```python
from build123d import *

# Parameters (mm, degrees)
SKETCH1_W          = 80
SKETCH1_H          = 15
SHELL2_T           = 1
SKETCH2_R          = 1
CUT_EXTRUDE1_DEPTH = 10
FILLET1_R          = 2


with BuildPart() as part:
    # Sketch1 → Revolve1 (revolve)
    with BuildSketch(Plane.XY, mode=Mode.PRIVATE) as revolve1_sk:
        with Locations((40, 7.5)):
            Rectangle(SKETCH1_W, SKETCH1_H)
    revolve(revolve1_sk.sketch.rotate(Axis((0, 0, 0), (1, 0, 0)), 90), axis=Axis((0, 0, 0), (1, 0, 0)))

    # Shell2 (no face opened: a closed hollow body)
    add(offset(amount=-SHELL2_T, mode=Mode.PRIVATE), mode=Mode.SUBTRACT)

    # Sketch2 → Cut-Extrude1 (cut)
    with BuildSketch(Plane(origin=(80, 0, 0), x_dir=(0, 0, -1), z_dir=(1, 0, 0))):
        Circle(SKETCH2_R)
    extrude(amount=-CUT_EXTRUDE1_DEPTH, mode=Mode.SUBTRACT)

    # Fillet1
    fillet1_edges = [part.edges().sort_by_distance(p)[0] for p in [
        (0, 0, -15),
        (80, 0, -15),
    ]]
    fillet(fillet1_edges, radius=FILLET1_R)


solid = part.part
```
CAD build for the part. Positions are in the model's coordinates, mm. A direction names the side the tool comes from. Coordinates: 2 decimals unless noted, no trailing zeros. Order: outer loops, then holes, each group sorted by start corner. A loop starts at its lowest first (then second) coordinate and runs counter-clockwise, first axis right, second up. Notation, with made-up numbers: (83.25, -39) - (139.25, -39) arc R24 ccw to (139.25, -22) - close; hole circle Ø8 at (45, 61). An arc over 180 degrees is marked (long way). Use a Markdown table: item, result. Add a question column.
(1) Drill centre lines: line 1 along X through (y, z) = (12.25, -2.25); line 2 along X through (y, z) = (0.25, 0.25); line 3 along Z through (x, y) = (68, -8). Where is each one in solid material? Low to high. Write a range as [from, to].
(2) Saw through at C-C (x = 71). Give the cut face in (y, z), then the cut area to 3 significant figures.
(3) Pull direction Z, two halves, no side cores. Call faces 1 (the face through (79.507, -0.976, 0.217)), 2 (the face through (0, 0, 0)), 3 (the face through (40.53, -12.65, 8.06)): +Z half, -Z half, draft (parallel to the pull), parting line (faces both ways), or undercut.
(4) Which spindle directions (+Z, -Z, +X, -X, +Y, -Y) get a long thin tool onto all of the face, cutting with end or side? Do faces 4 (the face through (80, 0, -3)), 5 (the face through (79, 3, 0)). Say none if no direction does.
(5) Saw through at A-A (z = 0). Give the cut face in (x, y), then the cut area to 3 significant figures.
(6) Flat gauge pins, fed straight in: pin 1 (1 mm diameter, centred on x = 57.5, z = 6.5, fed in from +Y); pin 2 (8 mm diameter, centred on x = 21, z = -5.5, fed in from -Y); pin 3 (1 mm diameter, centred on x = 40, y = 1, fed in from +Z). Where does each tip first touch, or does it go through?
Solved:
| question | item | result |
|---|---|---|
| 1 | line 1 | x = [0, 1], [79, 80] |
| 1 | line 2 | x = [0, 1] |
| 1 | line 3 | z = [-12.69, -11.49], [11.49, 12.69] |
| 2 | outline | circle Ø30 at (0, 0); hole circle Ø28 at (0, 0) |
| 2 | area | 91.1 mm² |
| 3 | face 1 | undercut |
| 3 | face 2 | draft |
| 3 | face 3 | parting line |
| 4 | face 4 | +Z, -Z, +X, +Y, -Y |
| 4 | face 5 | none |
| 5 | outline | (0, -13) arc R2 ccw to (2, -15) - (78, -15) arc R2 ccw to (80, -13) - (80, -1) - (79, -1) - (79, -14) - (1, -14) - (1, 14) - (79, 14) - (79, 1) - (80, 1) - (80, 13) arc R2 ccw to (78, 15) - (2, 15) arc R2 ccw to (0, 13) - close |
| 5 | area | 211 mm² |
| 6 | pin 1 | stops at y = 13.75 |
| 6 | pin 2 | stops at y = -14.92 |
| 6 | pin 3 | stops at z = 14.99 |
